Design review of the part shown in the three views and the two pictorial views. Dimensions are in mm from the part's minimum x, y and z. A direction names the side the tool comes from. Round coordinates to 2 decimals unless told otherwise and drop trailing zeros. Order: outer loops, then holes, each group sorted by start corner. A loop starts at its lowest first (then second) coordinate and runs counter-clockwise, first axis right, second up.
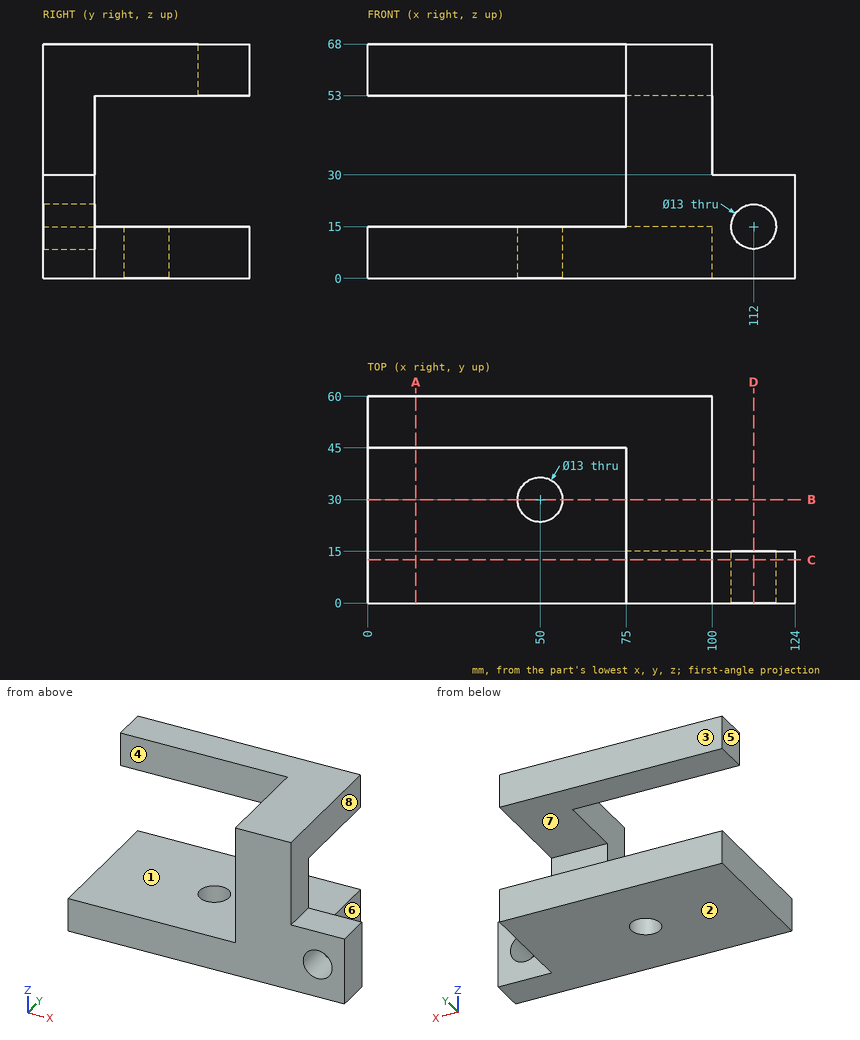
1) Take a section at B-B on y = 30. Give the boundary of the cut face in (x, z), plus the area to 3 significant figures.
Results:
outline: (0, 0) - (43.5, 0) - (43.5, 15) - (0, 15) - close; (56.5, 0) - (100, 0) - (100, 15) - (56.5, 15) - close; (75, 53) - (100, 53) - (100, 68) - (75, 68) - close
area: 1,680 mm2
2) Clearance check with flat-ended pins moving along their axes: P1, Ø3, axis at y = 11, z = 40.5, coming from the +X side; P2, Ø2, axis at x = 35.5, y = 27, coming from the +Z side; P3, Ø4.5, axis at x = 118, y = 8.5, coming from the +Z side; P4, Ø8, axis at x = 50, y = 30, coming from the +Z side. State where each tip first meets the part, or that it passes through.
Results:
P1: stops at x = 100
P2: stops at z = 15
P3: stops at z = 30
P4: passes through
3) To check wall thickness, follow line 1 along Z through (x, y) = (70, 53); line 2 along Y through (x, z) = (50, 10); line 3 along Z through (x, y) = (26.5, 6.5). State the ranges of each line that lie inside material, in increasing order.
Results:
line 1: z = 0 to 15, 53 to 68
line 2: y = 0 to 23.5, 36.5 to 60
line 3: z = 0 to 15
4) Take a section at C-C on y = 12.5. Give the boundary of the cut face in (x, z).
Results:
outline: (0, 0) - (124, 0) - (124, 30) - (100, 30) - (100, 68) - (75, 68) - (75, 15) - (0, 15) - close; hole circle Ø13 at (112, 15)
5) The part is to be moulded in two halves that separate along Z. For the marked faces 1, 2 and 3, say which applies: released by +Z, released by -Z, zero draft, split by the parting line, or undercut.
Results:
face 1: undercut
face 2: released by -Z
face 3: zero draft
6) For the marked faces 4, 5, 6, 7 and 8, list the 3-axis set-ups (+Z, -Z, +X, -X, +Y, -Y) from which the entire face can be reached by the end or side of a thin tool; tool diameter is ignored.
Results:
face 4: +Z, -X, -Y
face 5: +Z, -Z, -X, +Y, -Y
face 6: +Z, -Z, +X, +Y
face 7: +X, -X, +Y
face 8: +Z, +X, +Y, -Y
7) Take a section at A-A on x = 14. Give the boundary of the cut face in (y, z).
Results:
outline: (0, 0) - (60, 0) - (60, 15) - (0, 15) - close; (45, 53) - (60, 53) - (60, 68) - (45, 68) - close
8) Take a section at D-D on x = 112. Give the boundary of the cut face in (y, z).
Results:
outline: (0, 0) - (15, 0) - (15, 8.5) - (0, 8.5) - close; (0, 21.5) - (15, 21.5) - (15, 30) - (0, 30) - close
